Design review of the part built by this model. Coordinates are the model's own, in mm. A direction names the side the tool comes from. Coordinates: 2 decimals unless noted, no trailing zeros. Loops run counter-clockwise (first coordinate to the right, second up) from the corner with the lowest first, then second, coordinate; pieces in that order, holes last. Notation, with made-up numbers: M 48.25,-25.75 L 84.25,-25.75 A27 ccw 84.25,13.25 Z; hole C 62.25,6.25 d10. An arc over 180 degrees is marked long. Put each result on its own line as item: value. Start each with the question number.
(1) The part is to be moulded in two halves that separate along X. For faces 4 (the flat face through (28, -30, 0)), 5 (the cylindrical face through (59.046, -6.936, 3.815)), 6 (the flat face through (59.69, -19, 0)), say which applies: +X half, -X half, draft (parallel to the pull), parting line (faces both ways), or undercut.
(2) Take a section at D-D, the plane x = 14.5. Give the boundary of the cut face in (y, z), then the cut area to 3 significant figures.
(3) Take a section at B-B, the plane z = 8.75. Give the boundary of the cut face in (x, y).
(4) Take a section at A-A, the plane y = -31. Give the boundary of the cut face in (x, z), then the cut area to 3 significant figures.
(5) Take a section at C-C, the plane z = -8.5. Give the boundary of the cut face in (x, y).
(6) Clearance check with flat-ended pins moving along their axes: pin 1 (2 mm diameter, centred on x = 46, z = -3.5, fed in from -Y); pin 2 (3 mm diameter, centred on x = 26, y = -34, fed in from -Z). State where each tip first meets the part, or that it passes through.
(7) For faces 1 (the flat face through (-2.54, -16, -3)), 2 (the flat face through (28, -8, 0)), 3 (the cylindrical face through (-3.166, -31.164, 3.815)), list the 3-axis set-ups (+Z, -Z, +X, -X, +Y, -Y) from which the entire face can be reached by the end or side of a thin tool; tool diameter is ignored.
(8) For probe 1 along X at (y, z) = (-20, 6); probe 2 along X at (y, z) = (-15.5, -4.5); probe 3 along X at (y, z) = (-5, 11.25), list the stretches that pass through material, from the lowest coordinate up. Write a range as [from, to].
```python
from build123d import *

# Parameters (mm, degrees)
F0_W     = 55.88
F0_H     = 12.7
F1_DEPTH = 38.1
F3_DEPTH = 58.42
F2_R     = 3.81
F4_DEPTH = 2.54
F5_R     = 12.7
F6_DEPTH = 1.27
F7_R     = 12.7
F8_DEPTH = 1.27


with BuildPart() as f1:
    # F0 (on Front) → F1 (new body)
    with BuildSketch(Plane.XZ):
        with Locations((27.94, 6.35)):
            Rectangle(F0_W, F0_H)
    extrude(amount=F1_DEPTH)

    # F2 (on face) → F3 (join)
    with BuildSketch(Plane.YZ.offset(55.88)):
        with BuildLine():
            ThreePointArc((-22.86, 0), (-19.05, -3.81), (-15.24, 0))
            Line((-15.24, 0), (-22.86, 0))
        make_face()
        with BuildLine():
            Line((-22.86, 0), (-15.24, 0))
            ThreePointArc((-15.24, 0), (-19.05, 3.81), (-22.86, 0))
        make_face()
    extrude(amount=-F3_DEPTH)

    # F2 (on face) → F4 (join)
    with BuildSketch(Plane.YZ.offset(55.88)):
        with Locations((-19.05, 0)):
            Circle(F2_R)
    extrude(amount=F4_DEPTH)

    # F5 (on face) → F6 (join)
    with BuildSketch(Plane(origin=(-2.54, 0, 0), x_dir=(0, -1, 0), z_dir=(-1, 0, 0))):
        with Locations((19.05, 0)):
            Circle(F5_R)
    extrude(amount=F6_DEPTH)

    # F7 (on face) → F8 (join)
    with BuildSketch(Plane.YZ.offset(58.42)):
        with Locations((-19.05, 0)):
            Circle(F7_R)
    extrude(amount=F8_DEPTH)


solid = f1.part
```
Computed values:
1. face 4: undercut
1. face 5: draft
1. face 6: +X half
2. outline: M -38.1,0 L -22.86,0 A3.81 ccw -15.24,0 L 0,0 L 0,12.7 L -38.1,12.7 Z
2. area: 507 mm^2
3. outline: M -3.81,-28.25 L -2.54,-28.25 L -2.54,-9.85 L -3.81,-9.85 Z; M 0,-38.1 L 55.88,-38.1 L 55.88,0 L 0,0 Z; M 58.42,-28.25 L 59.69,-28.25 L 59.69,-9.85 L 58.42,-9.85 Z
4. outline: M -3.81,-4.3 L -2.54,-4.3 L -2.54,4.3 L -3.81,4.3 Z; M 0,0 L 55.88,0 L 55.88,12.7 L 0,12.7 Z; M 58.42,-4.3 L 59.69,-4.3 L 59.69,4.3 L 58.42,4.3 Z
4. area: 732 mm^2
5. outline: M -3.81,-28.49 L -2.54,-28.49 L -2.54,-9.61 L -3.81,-9.61 Z; M 58.42,-28.49 L 59.69,-28.49 L 59.69,-9.61 L 58.42,-9.61 Z
6. pin 1: stops at y = -21.93
6. pin 2: stops at z = 0
7. face 1: none
7. face 2: -Z, +Y
7. face 3: -X
8. probe 1: x = [-3.81, -2.54], [0, 55.88], [58.42, 59.69]
8. probe 2: x = [-3.81, -2.54], [58.42, 59.69]
8. probe 3: x = [0, 55.88]
